The model under review builds one solid part; all positions refer to its coordinate system, in mm. A direction names the side the tool comes from. Coordinates: 2 decimals unless noted, no trailing zeros. Write each loop counter-clockwise with the first axis right and the second up, starting at its lowest first coordinate (ties: lowest second). Pieces come first, ordered by that corner, then holes. Notation, with made-up numbers: (36, 85) -> (46, 85) arc R16 cw to (46, 105) -> close; hole circle Ø7 at (-21.75, 3). An arc over 180 degrees is marked (long way). Write each question's results on one line, items separated by ' | '.
```python
from build123d import *

# Parameters (mm, degrees)
SKETCH3_W = 6
SKETCH3_H = 1.45


with BuildPart() as part:
    # Sweep1: sweep along a path in Sketch2
    with BuildLine(Plane.XY) as sweep1_path:
        Line((2.67002525, -9.567055565), (-59.502854179, -26.918596678))
        ThreePointArc((-59.502854179, -26.918596678), (-66.944770348, -23.008271135), (-63.479166051, -15.349136134))
        Line((-63.479166051, -15.349136134), (-3.775591162, 9.187083237))
        ThreePointArc((-3.775591162, 9.187083237), (9.393348687, 3.228403239), (2.67002525, -9.567055565))
    # Sketch3 → Sweep1 (sweep)
    with BuildSketch(Plane(origin=(-63.479166051, -15.349136134, 0), x_dir=(0, 0, -1), z_dir=(0.9249375405656244, 0.38011912087188415, 0))):
        with Locations((0, 0.725)):
            Rectangle(SKETCH3_W, SKETCH3_H)
    sweep(path=sweep1_path.line)


solid = part.part
```
Q1. Clearance check with a flat-ended pin moving along its axis: P1, Ø3, axis at x = -4, z = -2, coming from the +Y side. State where the tip first meets the part, or that it passes through.
Solution:
P1: y = 11.1
Q2. Add section B-B (z = 1). Write out the cut boundary in (x, y), plus the area to 3 significant figures.
Solution:
outline: (-64.03, -14.01) arc R7.58 ccw to (-59.11, -28.32) -> (3.06, -10.96) arc R11.38 ccw (long way) to (-4.33, 10.53) -> close; hole (-63.48, -15.35) arc R6.13 ccw to (-59.5, -26.92) -> (2.67, -9.57) arc R9.93 ccw (long way) to (-3.78, 9.19) -> close | area: 268 mm²
Q3. Add section C-C (x = -32). Write out the cut boundary in (y, z).
Solution:
outline: (-20.75, -3) -> (-19.24, -3) -> (-19.24, 3) -> (-20.75, 3) -> close; (-2.41, -3) -> (-0.84, -3) -> (-0.84, 3) -> (-2.41, 3) -> close
Q4. For line 1 (Y direction, x = -59.5, z = 2); line 2 (X direction, y = 8, z = -2.25); line 3 (Y direction, x = -48, z = 1.75), list the stretches that pass through material, from the lowest coordinate up. Write a range as from..to.
Solution:
line 1: -28.41..-26.92, -13.71..-12.15 | line 2: -10.48..-6.66, 5.89..8.1 | line 3: -25.21..-23.71, -8.99..-7.42
Q5. Machinability: for faces 1 (the flat face through (-27, -19, -3)), 2 (the flat face through (-28.852, -18.364, 0.042)), which of the approach directions +Z, -Z, +X, -X, +Y, -Y give a long, thin tool a straight path to every point of the face, cutting with its end or side? Answer none if there is none.
Solution:
face 1: -Z, +X, -X, +Y, -Y | face 2: +Z, -Z
Q6. Add section A-A (y = 1). Write out the cut boundary in (x, z).
Solution:
outline: (-27.51, -3) -> (-23.7, -3) -> (-23.7, 3) -> (-27.51, 3) -> close; (9.88, -3) -> (11.34, -3) -> (11.34, 3) -> (9.88, 3) -> close
Q7. Draft analysis for pull direction X (two halves, no side actions). For faces 3 (the flat face through (-26.7, -18, 3)), 4 (the cylindrical face through (-66.9, -23.13, -0.04)), 5 (the flat face through (-33.76, -1.57, -0.04)), state which applies: pulls with the +X half, pulls with the -X half, needs draft (parallel to the pull), parting line crosses it, or undercut.
Solution:
face 3: needs draft | face 4: undercut | face 5: pulls with the -X half
